Source: CAD feature listing. Evaluate the final solid. Frame: model axes, mm. A direction names the side the tool comes from. Coordinates: 2 decimals unless noted, no trailing zeros. Loops run counter-clockwise (first coordinate to the right, second up) from the corner with the lowest first, then second, coordinate; pieces in that order, holes last. Notation, with made-up numbers: (-24, 23.5) - (23, 23.5) arc R11 ccw to (23, 36.5) - close; hole circle Ø3 at (-14, -19.5). An arc over 180 degrees is marked (long way). Use CSV: the item, a comma, the result in double quotes. Start each with the question number.
Autodesk Inventor part; units mm, degrees
ref_plane "YZ Plane" through (0, 0, 0) normal (1, 0, 0) x (0, 1, 0)
ref_plane "XZ Plane" through (0, 0, 0) normal (0, 1, 0) x (-1, 0, 0)
ref_plane "XY Plane" through (0, 0, 0) normal (0, 0, 1) x (1, 0, 0)
sketch "Sketch1" plane through (0, 0, 0) normal (0, 1, 0) x (-1, 0, 0)
  line L0 (-98, 30) -> (98, 30)
  line L1 (100, 28) -> (100, -28)
  line L2 (98, -30) -> (-98, -30)
  line L3 (-100, -28) -> (-100, 28)
  line L4 (-100, 30) -> (100, -30) construction
  line L5 (100, 30) -> (-100, -30) construction
  arc A0 (-98, 30) -> (-100, 28) centre (-98, 28) ccw
  arc A1 (100, 28) -> (98, 30) centre (98, 28) ccw
  arc A2 (98, -30) -> (100, -28) centre (98, -28) ccw
  arc A3 (-100, -28) -> (-98, -30) centre (-98, -28) ccw
  circle A4 centre (-22, 0) radius 22
  circle A5 centre (-50, 0) radius 3.75
  circle A6 centre (6, 0) radius 3.75
  circle A7 centre (30, 15) radius 3.25
  circle A8 centre (50, 15) radius 3.25
  circle A9 centre (70, 15) radius 3.25
  circle A10 centre (30, -15) radius 3.25
  circle A11 centre (50, -15) radius 3.25
  circle A12 centre (70, -15) radius 3.25
  point P0 (0, 0)
  point P1 (-100, 0)
  dimension "d0" = 60
  dimension "d1" = 200
  dimension "d2" = 2
  dimension "d3" = 44
  dimension "d4" = 56
  dimension "d5" = 28
  dimension "d6" = 7.5
  dimension "d7" = 7.5
  dimension "d8" = 50
  dimension "d9" = 6.5
  dimension "d10" = 6.5
  dimension "d11" = 6.5
  dimension "d12" = 6.5
  dimension "d13" = 6.5
  dimension "d14" = 6.5
  dimension "d15" = 15
  dimension "d16" = 30
  dimension "d17" = 30
  dimension "d18" = 20
  dimension "d19" = 20
extrude "Plate1" add sketch "Sketch1" along normal mid plane 10
sketch "Sketch2" plane through (0, 5, 0) normal (0, 1, 0) x (1, 0, 0)
  line L0 (98, -30) -> (-98, -30)
  line L1 (100, 30) -> (60, 30)
  line L2 (60, 30) -> (60, -30)
  line L3 (60, -30) -> (100, -30)
  line L4 (100, -30) -> (100, 30)
  line L5 (100, 28) -> (100, -28)
  line L6 (-98, 30) -> (98, 30)
  point P0 (0, 0)
  dimension "d21" = 40
extrude "Cut1" cut sketch "Sketch2" against normal blind 10
fillet "Corner Round1" radius 2 2 edges at (60, 0, -30) (60, 0, 30)
sketch "Sketch3" plane through (0, 5, 0) normal (0, 1, 0) x (1, 0, 0)
  line L0 (-98, 30) -> (58, 30) construction
  line L1 (-100, -28) -> (-100, 28) construction
  line L2 (-100, 30) -> (-80, 30)
  line L3 (-80, 30) -> (-80, -30)
  line L4 (-80, -30) -> (-100, -30)
  line L5 (-100, -30) -> (-100, 30)
  circle A0 centre (-70, -15) radius 3.25
  point P0 (0, 0)
  point P1 (-98, -30)
  dimension "d26" = 20
extrude "Cut2" cut sketch "Sketch3" against normal blind 10 contours L2 L3 L4 L5
sketch "Sketch4" plane through (0, 5, 0) normal (0, 1, 0) x (1, 0, 0)
  circle A0 centre (-70, 15) radius 3.25
  circle A1 centre (-50, 15) radius 3.25
  circle A2 centre (-30, 15) radius 3.25
  circle A3 centre (-30, -15) radius 3.25
  circle A4 centre (-50, -15) radius 3.25
  circle A5 centre (-70, -15) radius 3.25
  point P0 (0, 0)
hole "Hole1" at (-70, 5, -15) at (-50, 5, -15) at (-30, 5, -15) at (-30, 5, 15) at (-50, 5, 15) at (-70, 5, 15) direction (0, -1, 0) diameter 12 depth 6
equation "\"d7\" = d6"
equation "\"d10\" = d9"
equation "\"d11\" = d9"
equation "\"d12\" = d9"
equation "\"d13\" = d9"
equation "\"d14\" = d9"
equation "\"d22\" = Thickness"
equation "\"d27\" = Thickness"
equation "\"d20\" = Thickness"
equation "\"BendReliefDepth\" = 0.5 * Thickness"
properties part number "HCMUTE-CDT23-BAT_TRUC_DAN" material "Stainless Steel"
(1) Section A-A on x = 50. Output: boundary loops of the cut face in (y, z).
(2) Reachability of faces 1 (the cylindrical face through (-33.1, -3.03, -15.98)), 2 (the cylindrical face through (-47.7, 1.96, -9.46)) from +Z, -Z, +X, -X, +Y, -Y: full face, straight path, thin tool, end or side. Return the list, or none.
(3) Section B-B on x = -50. Output: boundary loops of the cut face in (y, z), plus the area to 3 significant figures.
(4) Pin query (flat end, axial travel): pin 1 Ø5 at (x, z) = (-70, 15) entering from +Y; pin 2 Ø6 at (x, z) = (-70.5, -16) entering from +Y. Return the tip coordinate at first contact, or that it passes through.
(5) Section C-C on z = -15. State how many separate pieces and enclosed holes the cut face has, plus the area to 3 significant figures.
(6) Draft query along Z for faces 3 (the flat face through (-9, 5, -6)), 4 (the flat face through (-10, 0, 30)), 5 (the flat face through (-27, -1, -12)), 6 (the cylindrical face through (-75.059, 1.958, 18.226)). Return one class per face: released by +Z, released by -Z, zero draft, split by the parting line, or undercut.
(7) Ray query, line 1 (Z direction, x = -30, y = 2.2); line 2 (X direction, y = 2.35, z = 15); line 3 (Z direction, x = -50, y = -2.6). Return the intervals inside material, ascending. Write a range as [from, to].
Solution:
1,outline,"(-5, -30) - (5, -30) - (5, -3.75) - (-5, -3.75) - close; (-5, 3.75) - (5, 3.75) - (5, 30) - (-5, 30) - close"
2,face 1,"+Y, -Y"
2,face 2,"+Y"
3,outline,"(-5, -30) - (5, -30) - (5, -21) - (-1, -21) - (-1, -18.25) - (-5, -18.25) - close; (-5, -11.75) - (-1, -11.75) - (-1, -9) - (5, -9) - (5, 9) - (-1, 9) - (-1, 11.75) - (-5, 11.75) - close; (-5, 18.25) - (-1, 18.25) - (-1, 21) - (5, 21) - (5, 30) - (-5, 30) - close"
3,area,"404 mm²"
4,pin 1,"passes through"
4,pin 2,"stops at y = -1"
5,separate pieces,"5"
5,enclosed holes,"0"
5,area,"784 mm²"
6,face 3,"zero draft"
6,face 4,"released by +Z"
6,face 5,"undercut"
6,face 6,"undercut"
7,line 1,"z = [-30, -21], [-9, 9], [21, 30]"
7,line 2,"x = [-80, -76], [-64, -56], [-44, -36], [-24, 5.91], [38.09, 60]"
7,line 3,"z = [-30, -18.25], [-11.75, 11.75], [18.25, 30]"
